Check sheet for the modelled part. Datum: model origin and axes. Units: mm. Round coordinates to 2 decimals unless told otherwise and drop trailing zeros. Loops run counter-clockwise (first coordinate to the right, second up) from the corner with the lowest first, then second, coordinate; pieces in that order, holes last. Notation, with made-up numbers: (22.25, -14) - (36.25, -14) arc R26 ccw to (36.25, 4) - close; hole circle Ø4 at (-24.5, -32.75). An arc over 180 degrees is marked (long way). Put each result on its own line as item: value.
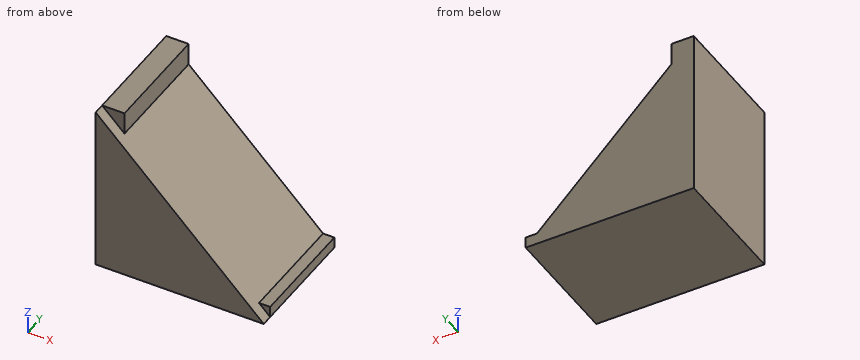
```python
from build123d import *

# Parameters (mm, degrees)
F1_W     = 20
F1_H     = 30
F2_DEPTH = 4
F4_DEPTH = 2
F5_E7_W  = 30
F5_E7_H  = 20
F6_DEPTH = 2
F7_DEPTH = 20


with BuildPart() as f2:
    # F1 (on Right) → F2 (new body)
    with BuildSketch(Plane.YZ):
        with Locations((10, 15)):
            Rectangle(F1_W, F1_H)
    extrude(amount=F2_DEPTH)

    # F0 (on Front) → F4 (join)
    with BuildSketch(Plane.XZ):
        Polygon((0, 30), (0, 0), (30, 0), align=None)
    extrude(amount=F4_DEPTH)

    # F5_E7 (on explicit) → F6 (join)
    with BuildSketch(Plane.XY):
        with Locations((15, 10)):
            Rectangle(F5_E7_W, F5_E7_H)
    extrude(amount=F6_DEPTH)

    # F7 (add): a face of the model
    f7_faces = [f2.faces().sort_by_distance(p)[0] for p in [
        (12, 0, 10),
    ]]
    extrude(f7_faces, amount=F7_DEPTH)


solid = f2.part
```
Item 1: Go/stop test with flat-tipped pins: pin 1 (2 mm diameter, centred on y = 8.5, z = 29, fed in from +X); pin 2 (2 mm diameter, centred on x = 20.5, y = 10.5, fed in from +Z); pin 3 (1 mm diameter, centred on x = 29.5, y = 8, fed in from +Z). Record where each tip stops, or that it passes through.
Filled sheet:
pin 1: x = 4
pin 2: z = 10.5
pin 3: z = 2
Item 2: Thickness scan on line 1 (X direction, y = 7.25, z = 26); line 2 (Z direction, x = 9, y = 15). Record the ranges inside material, lowest first. Write a range as from..to.
Filled sheet:
line 1: 0..4
line 2: 0..21
Item 3: Section check A-A on y = 9. Enter the section's corners in (x, z), then the cut area to 3 significant figures.
Filled sheet:
outline: (0, 0) - (30, 0) - (30, 2) - (28, 2) - (4, 26) - (4, 30) - (0, 30) - close
area: 460 mm²
Item 4: Section check B-B on z = 25.5. Enter the section's corners in (x, y), then the cut area to 3 significant figures.
Filled sheet:
outline: (0, -2) - (4.5, -2) - (4.5, 20) - (0, 20) - close
area: 99.0 mm²
Item 5: Section check C-C on x = 13. Enter the section's corners in (y, z), then the cut area to 3 significant figures.
Filled sheet:
outline: (-2, 0) - (20, 0) - (20, 17) - (-2, 17) - close
area: 374 mm²
